```python
from build123d import *

# Parameters (mm, degrees)
SKETCH1_W           = 150
SKETCH1_H           = 485
SKETCH1_W_2         = 345
SKETCH1_W_3         = 305
BOSS_EXTRUDE1_DEPTH = 2
SKETCH2_W           = 2010
SKETCH2_H           = 535
SKETCH2_W_2         = 2000
SKETCH2_H_2         = 525
BOSS_EXTRUDE2_DEPTH = 25
BOSS_EXTRUDE3_DEPTH = 80
SKETCH4_W           = 40
SKETCH4_H           = 150
BOSS_EXTRUDE4_DEPTH = 5
BOSS_EXTRUDE5_DEPTH = 80
SKETCH8_R           = 2
BOSS_EXTRUDE7_DEPTH = 20


with BuildPart() as part:
    # Sketch1 → Boss-Extrude1 (new body)
    with BuildSketch(Plane(origin=(0, 0, 0), x_dir=(1, 0, 0), z_dir=(0, 1, 0))):
        Polygon((1000, -262.5), (1000, 242.5), (1000, 262.5), (-1000, 262.5), (-1000, -262.5), align=None)
        with Locations((-905, 0)):
            Rectangle(SKETCH1_W, SKETCH1_H, mode=Mode.SUBTRACT)
        with Locations((-632.5, 0)):
            Rectangle(SKETCH1_W_2, SKETCH1_H, mode=Mode.SUBTRACT)
        with Locations((-262.5, 0)):
            Rectangle(SKETCH1_W_2, SKETCH1_H, mode=Mode.SUBTRACT)
        with Locations((107.5, 0)):
            Rectangle(SKETCH1_W_2, SKETCH1_H, mode=Mode.SUBTRACT)
        with Locations((827.5, 0)):
            Rectangle(SKETCH1_W_3, SKETCH1_H, mode=Mode.SUBTRACT)
        with Locations((477.5, 0)):
            Rectangle(SKETCH1_W_2, SKETCH1_H, mode=Mode.SUBTRACT)
    extrude(amount=BOSS_EXTRUDE1_DEPTH)

    # Sketch2 → Boss-Extrude2 (add)
    with BuildSketch(Plane(origin=(0, 0, 0), x_dir=(1, 0, 0), z_dir=(0, 1, 0))):
        Rectangle(SKETCH2_W, SKETCH2_H)
        Rectangle(SKETCH2_W_2, SKETCH2_H_2, mode=Mode.SUBTRACT)
    extrude(amount=BOSS_EXTRUDE2_DEPTH)

    # Sketch3 → Boss-Extrude3 (add)
    with BuildSketch(Plane(origin=(1005, 0, 0), x_dir=(0, 0, -1), z_dir=(1, 0, 0))):
        Polygon((-20, 25), (-20, 0), (20, 0), (20, 5), (-15, 5), (-15, 25), align=None)
    extrude(amount=BOSS_EXTRUDE3_DEPTH)

    # Sketch4 → Boss-Extrude4 (add)
    with BuildSketch(Plane(origin=(0, 0, 15), x_dir=(-1, 0, 0), z_dir=(0, 0, -1))):
        with Locations((-1065, 80)):
            Rectangle(SKETCH4_W, SKETCH4_H)
    extrude(amount=BOSS_EXTRUDE4_DEPTH)

    # Sketch5 → Boss-Extrude5 (add)
    with BuildSketch(Plane.ZY.offset(1005)):
        Polygon((15, 25), (15, 0), (-15, 0), (-15, 5), (10, 5), (10, 25), align=None)
    extrude(amount=BOSS_EXTRUDE5_DEPTH)

    # Sketch8 → Boss-Extrude7 (add)
    with BuildSketch(Plane.XY.offset(15)):
        with Locations((-1077, 12.5)):
            Circle(SKETCH8_R)
    extrude(amount=-BOSS_EXTRUDE7_DEPTH)


solid = part.part
```
Can you work these out from the model? Positions are in its coordinate system, mm. Coordinates: 2 decimals unless noted, no trailing zeros. Order: outer loops, then holes, each group sorted by start corner. A loop starts at its lowest first (then second) coordinate and runs counter-clockwise, first axis right, second up. Notation, with made-up numbers: (61.5, -33) - (72.5, -33) arc R16 cw to (72.5, -28) - close; hole circle Ø6 at (36, 20.5). An arc over 180 degrees is marked (long way). Answer in a Markdown table with one row per item.
1. Suppose I cut it at C-C (y = 79.5). Please give me the cut outline in (x, z).
Reply:
| item | result |
|---|---|
| outline | (1045, 10) - (1085, 10) - (1085, 15) - (1045, 15) - close |
2. For pin 1 (7.5 mm diameter, centred on x = 1033, y = 16, fed in from +Z); pin 2 (0.6 mm diameter, centred on y = 0.5, z = -80.5, fed in from -X); pin 3 (12.5 mm diameter, centred on x = -1034.5, y = 15, fed in from +Z), each with a flat end and sliding along its axis, tell me the tip position at first contact or that it passes through.
Reply:
| item | result |
|---|---|
| pin 1 | stops at z = 20 |
| pin 2 | stops at x = -1005 |
| pin 3 | stops at z = 15 |
3. Suppose I cut it at B-B (x = -346.5). Please give me the cut outline in (y, z).
Reply:
| item | result |
|---|---|
| outline | (0, -267.5) - (25, -267.5) - (25, -262.5) - (2, -262.5) - (2, -242.5) - (0, -242.5) - close; (0, 242.5) - (2, 242.5) - (2, 262.5) - (25, 262.5) - (25, 267.5) - (0, 267.5) - close |
4. If we mould it in two halves opening along Z, with no side actions, what happens to faces 1 (the flat face through (-79, 2, -21)), 2 (the flat face through (1044, 5, -3)), 3 (the flat face through (1065, 91, 15)), 4 (the flat face through (1065, 81, 10))? For each: pulls with the +Z half, pulls with the -Z half, needs draft (parallel to the pull), parting line crosses it, or undercut.
Reply:
| item | result |
|---|---|
| face 1 | undercut |
| face 2 | needs draft |
| face 3 | pulls with the +Z half |
| face 4 | pulls with the -Z half |
5. If I drill on line 1 along X through (y, z) = (20.5, 35.5); line 2 along Y through (x, z) = (664.5, -188.5); line 3 along X through (y, z) = (55, 14), over which ranges is the centre line in solid material (lowest first)?
Reply:
| item | result |
|---|---|
| line 1 | x = -1005 to -1000, 1000 to 1005 |
| line 2 | y = 0 to 2 |
| line 3 | x = 1045 to 1085 |
6. Suppose I cut it at A-A (z = -40.5). Give the number of separate pieces and of enclosed holes in the cut face, and give its area (3 significant figures).
Reply:
| item | result |
|---|---|
| separate pieces | 7 |
| enclosed holes | 0 |
| area | 580 mm^2 |
